```python
from build123d import *

# Parameters (mm, degrees)
F0_W      = 20
F0_H      = 20
F1_DEPTH  = 1
F2_R      = 1
F3_R      = 0.15
F6_W      = 20
F6_H      = 20
F6_R      = 0.15
F7_DEPTH  = 1
F8_D      = 2.5
F10_DEPTH = 0.2


with BuildPart() as f1:
    # F0 (on Top) → F1 (new body)
    with BuildSketch(Plane.XY):
        Rectangle(F0_W, F0_H)
    extrude(amount=-F1_DEPTH)

    # F2 (on face) → F4 section 0
    with BuildSketch(Plane.XY):
        Circle(F2_R)
    # F3 (on face) → F4 section 1
    with BuildSketch(Plane(origin=(0, 0, -1), x_dir=(1, 0, 0), z_dir=(0, 0, -1))):
        Circle(F3_R)
    loft(mode=Mode.SUBTRACT)

    # F6 (on face) → F7 (join)
    with BuildSketch(Plane(origin=(0, 0, -1), x_dir=(1, 0, 0), z_dir=(0, 0, -1))):
        Rectangle(F6_W, F6_H)
        Circle(F6_R, mode=Mode.SUBTRACT)
    extrude(amount=F7_DEPTH)

    # F8 (through all)
    with Locations(Plane.XY):
        with Locations((-7, -7), (7, -7), (7, 7), (-7, 7)):
            Hole(F8_D / 2)

    # F9 (on face) → F10 (join)
    with BuildSketch(Plane.XY):
        Polygon((-4.3009618943, -0.75), (-5.6, 1.5), (-6.8990381057, -0.75), align=None)
    extrude(amount=F10_DEPTH)


solid = f1.part
```
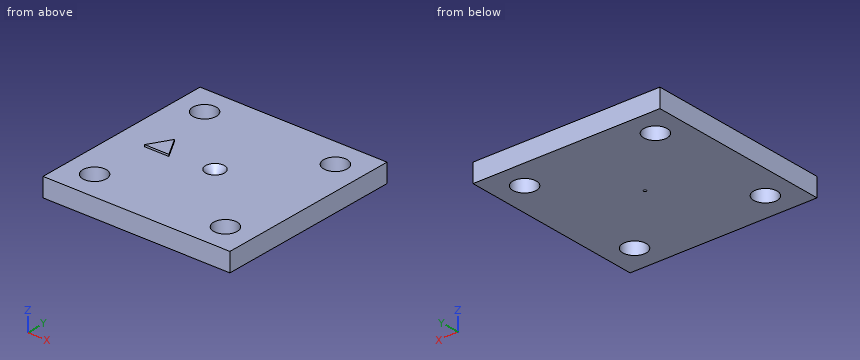
Model file for the job. Use its own axes, mm. Coordinates: 2 decimals unless noted, no trailing zeros. Order: outer loops, then holes, each group sorted by start corner. A loop starts at its lowest first (then second) coordinate and runs counter-clockwise, first axis right, second up. Notation, with made-up numbers: (-31, 37) -> (2, 37) arc R12 ccw to (2, 51) -> close; hole circle Ø1 at (3, 73.5). An arc over 180 degrees is marked (long way). Answer as a JSON object with one key per item and string values. Group by question number.
1) Flat gauge pins, fed straight in: pin 1 (3 mm diameter, centred on x = -7, y = -7, fed in from +Z); pin 2 (3 mm diameter, centred on x = 7, y = -7, fed in from -Z). Where does each tip first touch, or does it go through?
2) Drill centre lines: L1, parallel to Y at x = -7, z = -1.5; L2, parallel to X at y = 7.5, z = -0.8; L3, parallel to Y at x = -8, z = -1.5. Where is each one in solid material? Low to high.
3) Cut at C-C, the plane z = -1.25. Write the cut outline in (x, y), then the cut area to 3 significant figures.
4) Cut at D-D, the plane x = -6. Write the cut outline in (y, z), then the cut area to 3 significant figures.
5) Cut at A-A, the plane y = -7. Write the cut outline in (x, z), then the cut area to 3 significant figures.
Check values:
{
 "1": {"pin 1": "stops at z = 0", "pin 2": "stops at z = -2"},
 "2": {"L1": "y = -10 to -8.25, -5.75 to 5.75, 8.25 to 10", "L2": "x = -10 to -8.15, -5.85 to 5.85, 8.15 to 10", "L3": "y = -10 to -7.75, -6.25 to 6.25, 7.75 to 10"},
 "3": {"outline": "(-10, -10) -> (10, -10) -> (10, 10) -> (-10, 10) -> close; hole circle Ø2.5 at (-7, -7); hole circle Ø2.5 at (-7, 7); hole circle Ø0.3 at (0, 0); hole circle Ø2.5 at (7, -7); hole circle Ø2.5 at (7, 7)", "area": "380 mm²"},
 "4": {"outline": "(-10, -2) -> (-7.75, -2) -> (-7.75, 0) -> (-10, 0) -> close; (-6.25, -2) -> (6.25, -2) -> (6.25, 0) -> (0.81, 0) -> (0.81, 0.2) -> (-0.75, 0.2) -> (-0.75, 0) -> (-6.25, 0) -> close; (7.75, -2) -> (10, -2) -> (10, 0) -> (7.75, 0) -> close", "area": "34.3 mm²"},
 "5": {"outline": "(-10, -2) -> (-8.25, -2) -> (-8.25, 0) -> (-10, 0) -> close; (-5.75, -2) -> (5.75, -2) -> (5.75, 0) -> (-5.75, 0) -> close; (8.25, -2) -> (10, -2) -> (10, 0) -> (8.25, 0) -> close", "area": "30.0 mm²"}
}
